Autodesk Inventor part; units mm, degrees
ref_plane "YZ Plane" through (0, 0, 0) normal (1, 0, 0) x (0, 1, 0)
ref_plane "XZ Plane" through (0, 0, 0) normal (0, 1, 0) x (-1, 0, 0)
ref_plane "XY Plane" through (0, 0, 0) normal (0, 0, 1) x (1, 0, 0)
sketch "スケッチ1" plane through (0, 0, 0) normal (0, 0, 1) x (1, 0, 0)
  line L0 (0, 0) -> (190, 0)
  line L1 (190, 0) -> (190, 305)
  line L2 (190, 305) -> (0, 305)
  line L3 (0, 305) -> (0, 0)
  line L4 (0, 305) -> (40, 305)
  line L5 (40, 305) -> (40, 0)
  line L6 (40, 0) -> (0, 0)
  line L7 (0, 0) -> (0, 305)
  line L8 (190, 0) -> (150, 0)
  line L9 (150, 0) -> (150, 305)
  line L10 (150, 305) -> (190, 305)
  line L11 (190, 305) -> (190, 0)
  line L12 (0, 305) -> (190, 305)
  line L13 (190, 305) -> (190, 265)
  line L14 (190, 265) -> (0, 265)
  line L15 (0, 265) -> (0, 305)
  point P0 (40, 265)
  point P1 (150, 265)
  dimension "d0" = 305
  dimension "d1" = 190
  dimension "d2" = 40
  dimension "d3" = 40
  dimension "d4" = 40
extrude "押し出し1" add sketch "スケッチ1" along normal blind 30 contours L3 L14 L5 L0 | L3 L2 L5 L14 | L9 L14 L1 L0 | L5 L2 L9 L14 | L9 L2 L1 L14
fillet "フィレット1" radius 10 8 edges at (0, 305, 15) (0, 0, 15) (190, 305, 15) (40, 265, 15) (150, 265, 15) (150, 0, 15) (190, 0, 15) (40, 0, 15)
equation "\"d3\" = d2"
equation "\"d4\" = d2"
properties part number "BP_cover"
Work out the finished part from the listing and answer in its coordinate system (mm). A direction names the side the tool comes from. Round coordinates to 2 decimals unless told otherwise and drop trailing zeros. Loops run counter-clockwise (first coordinate to the right, second up) from the corner with the lowest first, then second, coordinate; pieces in that order, holes last.
(1) Find the intervals of material crossed by L1, parallel to X at y = 222, z = 1.75; L2, parallel to X at y = 257, z = 16.5; L3, parallel to Y at x = 88, z = 16.25, in increasing order.
Computed values:
L1: x = 0 to 40, 150 to 190
L2: x = 0 to 40.2, 149.8 to 190
L3: y = 265 to 305
(2) The part is cut by section C-C, the plane x = 88. Give the vertices of the cut face in (y, z).
Computed values:
outline: (265, 0) - (305, 0) - (305, 30) - (265, 30) - close
(3) The part is cut by section B-B, the plane z = 10.5. Give the vertices of the cut face in (x, y).
Computed values:
outline: (0, 10) arc R10 ccw to (10, 0) - (30, 0) arc R10 ccw to (40, 10) - (40, 255) arc R10 cw to (50, 265) - (140, 265) arc R10 cw to (150, 255) - (150, 10) arc R10 ccw to (160, 0) - (180, 0) arc R10 ccw to (190, 10) - (190, 295) arc R10 ccw to (180, 305) - (10, 305) arc R10 ccw to (0, 295) - close
(4) This flat-tipped pin is pushed along its axis until it touches: P1, Ø15, axis at x = 110, z = 15.5, coming from the -Y side. Where does it stop, or does it pass through?
Computed values:
P1: stops at y = 265
(5) For faces 5 (the flat face through (40, 134, 15)), 6 (the cylindrical face through (186.99, 2.85, 15.21)), determine the directions among +Z, -Z, +X, -X, +Y, -Y from which every point of the face is accessible in a straight line to the end or side of a thin tool.
Computed values:
face 5: +Z, -Z, -Y
face 6: +Z, -Z, +X, -Y
(6) The mould has two halves that part along X. Classify faces 1 (the cylindrical face through (2.85, 3.01, 15.21)), 2 (the cylindrical face through (187.15, 301.99, 15.21)), 3 (the flat face through (170, 0, 15)), 4 (the cylindrical face through (36.99, 2.85, 15.21)): pulls with the +X half, pulls with the -X half, needs draft (parallel to the pull), parting line crosses it, or undercut.
Computed values:
face 1: pulls with the -X half
face 2: pulls with the +X half
face 3: needs draft
face 4: undercut
(7) The part is cut by section A-A, the plane y = 56. Give the vertices of the cut face in (x, z), and give its area (3 significant figures).
Computed values:
outline: (0, 0) - (40, 0) - (40, 30) - (0, 30) - close; (150, 0) - (190, 0) - (190, 30) - (150, 30) - close
area: 2,400 mm2
